The listing builds one solid part. Answer for the finished solid, in the listing's coordinates (mm). A direction names the side the tool comes from. Coordinates: 2 decimals unless noted, no trailing zeros. Loops run counter-clockwise (first coordinate to the right, second up) from the corner with the lowest first, then second, coordinate; pieces in that order, holes last. Notation, with made-up numbers: (11, 57) - (55, 57) arc R32 cw to (55, 87) - close; hole circle Ø3 at (35, -17). An arc over 180 degrees is marked (long way). One line per question, with ' | ' between items.
from build123d import *

# Parameters (mm, degrees)
SKETCH_1_R          = 3.5
EXTRUDE_1_DEPTH     = 13
EXTRUDE_2_DEPTH     = 2
CUT_EXTRUDE_1_DEPTH = 13
SKETCH_4_R          = 1.25
CUT_EXTRUDE_2_DEPTH = 8
FILLET_1_R          = 1


with BuildPart() as part:
    # 草图1 → 凸台-拉伸1 (new body)
    with BuildSketch(Plane.XY):
        Circle(SKETCH_1_R)
    extrude(amount=EXTRUDE_1_DEPTH)

    # 草图2 → 凸台-拉伸2 (add)
    with BuildSketch(Plane.XY.offset(13)):
        with BuildLine():
            Line((-3.895324597, -0.909090909), (-1.460746724, -11.340909091))
            ThreePointArc((-1.460746724, -11.340909091), (0, -12.5), (1.460746724, -11.340909091))
            Line((1.460746724, -11.340909091), (3.895324597, -0.909090909))
            ThreePointArc((3.895324597, -0.909090909), (0, 4), (-3.895324597, -0.909090909))
        make_face()
    extrude(amount=EXTRUDE_2_DEPTH)

    # 草图3 → 切除-拉伸1 (cut)
    with BuildSketch(Plane(origin=(0, 0, 0), x_dir=(-1, 0, 0), z_dir=(0, 0, -1))):
        Polygon((0, 3.5), (-3.031088913, -1.75), (-6.759949263, -1.75), (0, 7.742275781), (6.759949263, -1.75), (3.031088913, -1.75), align=None)
    extrude(amount=-CUT_EXTRUDE_1_DEPTH, mode=Mode.SUBTRACT)

    # 草图4 → 切除-拉伸2 (cut)
    with BuildSketch(Plane(origin=(0, 0, 0), x_dir=(-1, 0, 0), z_dir=(0, 0, -1))):
        Circle(SKETCH_4_R)
    extrude(amount=-CUT_EXTRUDE_2_DEPTH, mode=Mode.SUBTRACT)

    # 圆角1
    fillet_1_edges = [part.edges().sort_by_distance(p)[0] for p in [
        (0, 3.5, 6.5),
    ]]
    fillet(fillet_1_edges, radius=FILLET_1_R)


solid = part.part
Item 1: Find section B-B, the plane z = 6. Write down the section's boundary in (x, y), plus the area to 3 significant figures.
Taken from the geometry:
outline: (-3.03, -1.75) arc R3.5 ccw to (3.03, -1.75) - (0.87, 2) arc R1 ccw to (-0.87, 2) - close; hole circle Ø2.5 at (0, 0) | area: 17.8 mm2
Item 2: Each of these flat-tipped pins is pushed along its axis until it touches: pin 1 Ø4 at (y, z) = (-4, 10.5) entering from +X; pin 2 Ø3 at (x, z) = (-3, 9) entering from +Y; pin 3 Ø2 at (x, z) = (-1, 4) entering from -Y. Where does it stop, or does it pass through?
Taken from the geometry:
pin 1: stops at x = 2.87 | pin 2: stops at y = 0.9 | pin 3: stops at y = -3.5
Item 3: Find section A-A, the plane x = 0. Write down the section's boundary in (y, z), plus the area to 3 significant figures.
Taken from the geometry:
outline: (-12.5, 13) - (-3.5, 13) - (-3.5, 0) - (-1.25, 0) - (-1.25, 8) - (1.25, 8) - (1.25, 0) - (2.5, 0) - (2.5, 13) - (4, 13) - (4, 15) - (-12.5, 15) - close | area: 91.0 mm2
Item 4: Find section D-D, the plane z = 12. Write down the section's boundary in (x, y).
Taken from the geometry:
outline: (-3.03, -1.75) arc R3.5 ccw to (3.03, -1.75) - (0.87, 2) arc R1 ccw to (-0.87, 2) - close
Item 5: Which of the six approach directions +Z, -Z, +X, -X, +Y, -Y give full straight-line access (tool end or side, diameter ignored) to faces 4 (the face through (1.933, 0.151, 6.409)), 5 (the face through (-1.964, 0.099, 6.409)), 6 (the face through (0, -4, 13)), 7 (the face through (-0.1, -3.5, 6.4))?
Taken from the geometry:
face 4: -Z, +X, +Y | face 5: -Z, -X, +Y | face 6: -Z | face 7: -Z, -Y
Item 6: The mould has two halves that part along X. Classify faces 1 (the face through (0.27, -1.22, 3.94)), 2 (the face through (2.66, -6.2, 13.99)), 3 (the face through (0, 2.5, 6.6)): pulls with the +X half, pulls with the -X half, needs draft (parallel to the pull), parting line crosses it, or undercut.
Taken from the geometry:
face 1: undercut | face 2: pulls with the +X half | face 3: parting line crosses it
Item 7: Find section C-C, the plane y = 1.75. Write down the section's boundary in (x, z).
Taken from the geometry:
outline: (-3.6, 13) - (-1.01, 13) - (-1.01, 0) - (1.01, 0) - (1.01, 13) - (3.6, 13) - (3.6, 15) - (-3.6, 15) - close
Item 8: Find the intervals of material crossed by line 1 (Y direction, x = 0, z = 6); line 2 (Z direction, x = 1.5, y = 1.5); line 3 (Z direction, x = 0, y = -0.25), in increasing order. Write a range as [from, to].
Taken from the geometry:
line 1: y = [-3.5, -1.25], [1.25, 2.5] | line 2: z = [13, 15] | line 3: z = [8, 15]
